Geometry check sheet. Reference: the model listing, model coordinates, mm. Coordinates: 2 decimals unless noted, no trailing zeros. Loops run counter-clockwise (first coordinate to the right, second up) from the corner with the lowest first, then second, coordinate; pieces in that order, holes last.
from build123d import *

# Parameters (mm, degrees)
SKETCH_1_W      = 135
SKETCH_1_H      = 35
EXTRUDE_1_DEPTH = 80
FILLET_1_R      = 10


with BuildPart() as part:
    # 草图1 → 凸台-拉伸1 (new body)
    with BuildSketch(Plane.XY):
        with Locations((67.5, 17.5)):
            Rectangle(SKETCH_1_W, SKETCH_1_H)
    extrude(amount=EXTRUDE_1_DEPTH)

    # 圆角1
    fillet_1_edges = [part.edges().sort_by_distance(p)[0] for p in [
        (0, 35, 40),
        (135, 35, 40),
        (135, 0, 40),
        (0, 0, 40),
    ]]
    fillet(fillet_1_edges, radius=FILLET_1_R)


solid = part.part
(1) Sectioned sample at B-B on y = 2. Record the cut outline in (x, z), and give its area (3 significant figures).
Findings:
outline: (4, 0) - (131, 0) - (131, 80) - (4, 80) - close
area: 10,200 mm2
(2) Sectioned sample at A-A on z = 16. Record the cut outline in (x, y), and give its area (3 significant figures).
Findings:
outline: (0, 10) arc R10 ccw to (10, 0) - (125, 0) arc R10 ccw to (135, 10) - (135, 25) arc R10 ccw to (125, 35) - (10, 35) arc R10 ccw to (0, 25) - close
area: 4,640 mm2
(3) Scan lines: L1, parallel to X at y = 27.5, z = 13.5; L2, parallel to X at y = 29.5, z = 61.5; L3, parallel to Y at x = 126, z = 6.5. Record each from-to range of solid material in increasing order.
Findings:
L1: x = 0.32 to 134.68
L2: x = 1.07 to 133.93
L3: y = 0.05 to 34.95
